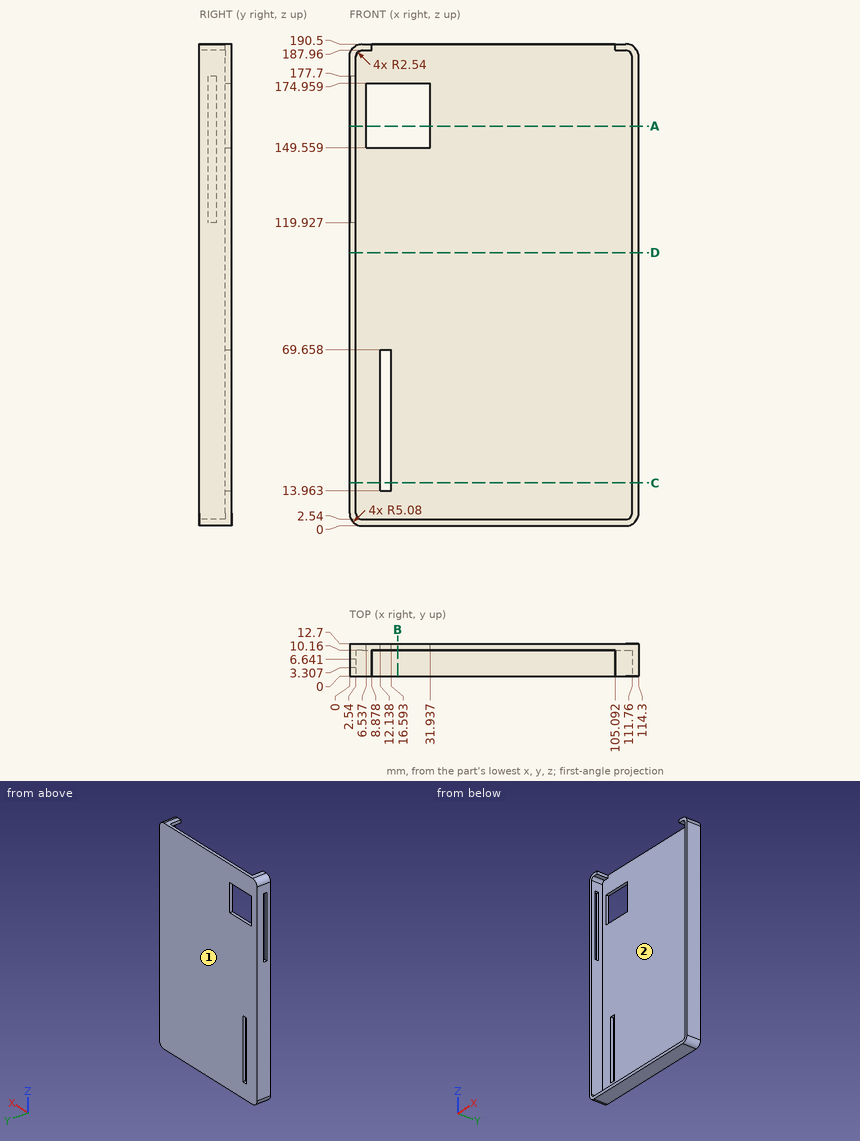
Answer from the drawing. Dimensions are ordinates in mm from the lowest x, y and z of the part. Give positions to 0.01 mm unless a question says otherwise; leave off trailing zeros. Order: outer loops, then holes, each group sorted by start corner. A loop starts at its lowest first (then second) coordinate and runs counter-clockwise, first axis right, second up. Notation, with made-up numbers: (60.5, 34) -> (86.5, 34) arc R7 ccw to (86.5, 41) -> close; hole circle Ø1 at (-4.75, 68). An arc over 180 degrees is marked (long way). Answer as a JSON object with one key per item and string values. Group by question number.
1. Flat-ended cylindrical pins translate along their axes: pin 1 Ø0.8 at (x, y) = (1.5, 5.5) entering from -Z; pin 2 Ø0.8 at (y, z) = (3.5, 188.5) entering from -X (1 decimal); pin 3 Ø3 at (x, y) = (36, 5) entering from +Z. Find the tip coordinate at first contact, or state that the pin passes through.
2. Consider line 1 along X through (y, z) = (9, 24.5); line 2 along Y through (x, z) = (86, 141.5); line 3 along X through (y, z) = (5.25, 165). Determine where each line is inside the solid, lowest interval first. Write a range as [from, to].
3. Section A-A on z = 158 is taken. Determine the outline of the cut face in (x, y).
4. Section B-B on x = 19 is taken. Determine the outline of the cut face in (y, z).
5. The mould has two halves that part along X. Classify the marked faces 1 and 2: released by +X, released by -X, zero draft, split by the parting line, or undercut.
6. Section D-D on z = 108 is taken. Determine the outline of the cut face in (x, y).
7. Section C-C on z = 17 is taken. Determine the outline of the cut face in (x, y).
Result sheet:
{
 "1": {"pin 1": "stops at z = 1.12", "pin 2": "stops at x = 0.8", "pin 3": "stops at z = 2.54"},
 "2": {"line 1": "x = [0, 2.54], [111.76, 114.3]", "line 2": "y = [10.16, 12.7]", "line 3": "x = [111.76, 114.3]"},
 "3": {"outline": "(0, 0) -> (2.54, 0) -> (2.54, 3.31) -> (0, 3.31) -> close; (0, 6.64) -> (2.54, 6.64) -> (2.54, 10.16) -> (6.54, 10.16) -> (6.54, 12.7) -> (0, 12.7) -> close; (31.94, 10.16) -> (111.76, 10.16) -> (111.76, 0) -> (114.3, 0) -> (114.3, 12.7) -> (31.94, 12.7) -> close"},
 "4": {"outline": "(0, 0) -> (12.7, 0) -> (12.7, 149.56) -> (10.16, 149.56) -> (10.16, 2.54) -> (0, 2.54) -> close; (10.16, 174.96) -> (12.7, 174.96) -> (12.7, 190.5) -> (10.16, 190.5) -> close"},
 "5": {"face 1": "zero draft", "face 2": "undercut"},
 "6": {"outline": "(0, 0) -> (2.54, 0) -> (2.54, 10.16) -> (111.76, 10.16) -> (111.76, 0) -> (114.3, 0) -> (114.3, 12.7) -> (0, 12.7) -> close"},
 "7": {"outline": "(0, 0) -> (2.54, 0) -> (2.54, 10.16) -> (12.14, 10.16) -> (12.14, 12.7) -> (0, 12.7) -> close; (16.59, 10.16) -> (111.76, 10.16) -> (111.76, 0) -> (114.3, 0) -> (114.3, 12.7) -> (16.59, 12.7) -> close"}
}
